Work out the finished part from the listing and answer in its coordinate system (mm). Face numbers are marked on the shaded views. Round coordinates to 2 decimals unless told otherwise and drop trailing zeros. Write each loop counter-clockwise with the first axis right and the second up, starting at its lowest first coordinate (ties: lowest second). Pieces come first, ordered by that corner, then holes.
1. Find section C-C (y = 10.5). Write down the section's boundary in (x, z), and give its area (3 significant figures).
2. Find section B-B (x = -10.5). Write down the section's boundary in (y, z) (3 decimals), and give its area (3 significant figures).
3. Determine the mould class of the marked faces 1, 2 and 3 for opening direction X: pulls with the +X half, pulls with the -X half, needs draft (parallel to the pull), parting line crosses it, or undercut.
4. Straight lines are drawn through the part: probe 1 along X at (y, z) = (3, 4); probe 2 along Z at (x, y) = (-4, 1.5); probe 3 along Z at (x, y) = (-4, 3.5). For each, find the intervals that lie inside material, in ascending order.
5. Find section A-A (y = 4.5). Write down the section's boundary in (x, z).
6. Flat-ended cylindrical pins translate along their axes: pin 1 Ø14.5 at (x, y) = (-3, 11) entering from +Z; pin 2 Ø1 at (x, z) = (10.5, 5) entering from +Y; pin 3 Ø3 at (x, z) = (-4, 4) entering from -Y. Find the tip coordinate at first contact, or state that the pin passes through.
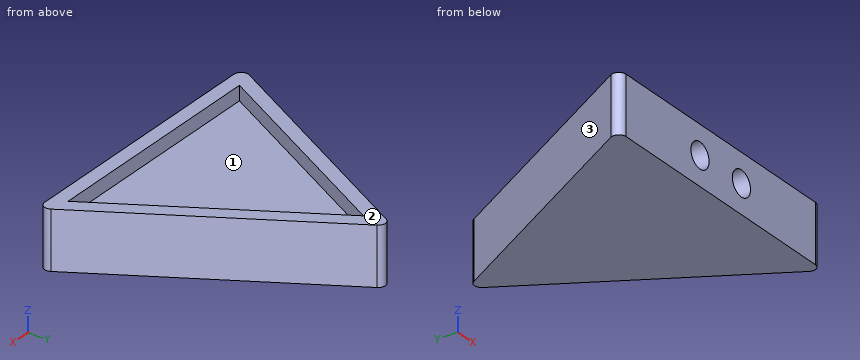
```python
from build123d import *

# Parameters (mm, degrees)
F1_DEPTH = 8
F3_DEPTH = 2
F5_D     = 3.5
F5_DEPTH = 8
F5_TIP   = 1.0515060833
F6_R     = 1


with BuildPart() as f1:
    # F0 (on Top) → F1 (new body)
    with BuildSketch(Plane.XY):
        Polygon((0, 35), (-20, 0), (20, 0), align=None)
    extrude(amount=F1_DEPTH)

    # F2 (on face) → F3 (cut)
    with BuildSketch(Plane.XY.offset(8)):
        Polygon((0, 30.9688711259), (-16.5536406433, 2), (16.5536406433, 2), align=None)
    extrude(amount=-F3_DEPTH, mode=Mode.SUBTRACT)

    # F5
    with Locations(Plane.XZ):
        with Locations((-4, 4), (4, 4)):
            Hole(F5_D / 2, depth=F5_DEPTH)
            with Locations((0, 0, -(F5_DEPTH + F5_TIP / 2))):  # 118° drill point
                Cone(0, F5_D / 2, F5_TIP, mode=Mode.SUBTRACT)

    # F6
    f6_edges = [f1.edges().sort_by_distance(p)[0] for p in [
        (0, 35, 4),
        (-20, 0, 4),
        (20, 0, 4),
    ]]
    fillet(f6_edges, radius=F6_R)


solid = f1.part
```
Worked answers:
1. outline: (-14, 0) - (14, 0) - (14, 8) - (11.7, 8) - (11.7, 6) - (-11.7, 6) - (-11.7, 8) - (-14, 8) - close
1. area: 177 mm2
2. outline: (0, 0) - (16.625, 0) - (16.625, 8) - (12.594, 8) - (12.594, 6) - (2, 6) - (2, 8) - (0, 8) - close
2. area: 112 mm2
3. face 1: undercut
3. face 2: needs draft
3. face 3: pulls with the -X half
4. probe 1: x = -18.29 to -5.75, -2.25 to 2.25, 5.75 to 18.29
4. probe 2: z = 0 to 2.25, 5.75 to 8
4. probe 3: z = 0 to 2.25, 5.75 to 6
5. outline: (-17.43, 0) - (17.43, 0) - (17.43, 8) - (15.13, 8) - (15.13, 6) - (-15.13, 6) - (-15.13, 8) - (-17.43, 8) - close; hole circle Ø3.5 at (-4, 4); hole circle Ø3.5 at (4, 4)
6. pin 1: stops at z = 6
6. pin 2: stops at y = 17.5
6. pin 3: stops at y = 8.15
